The model under review builds one solid part; all positions refer to its coordinate system, in mm. Face numbers are marked on the shaded views. A direction names the side the tool comes from. Coordinates: 2 decimals unless noted, no trailing zeros. Write each loop counter-clockwise with the first axis right and the second up, starting at its lowest first coordinate (ties: lowest second). Pieces come first, ordered by that corner, then holes.
1) For line 1 (Z direction, x = -4.5, y = 3.3); line 2 (X direction, y = 2.3, z = 19.5); line 3 (Z direction, x = -40.5, y = -15.5), list the stretches that pass through material, from the lowest coordinate up.
2) Machinability: for the marked faces 4 and 5, which of the approach directions +Z, -Z, +X, -X, +Y, -Y give a long, thin tool a straight path to every point of the face, cutting with its end or side? Answer none if there is none.
3) For P1, Ø16, axis at x = 5, z = 23, coming from the -Y side; P2, Ø12, axis at x = -50, z = 31, coming from the -Y side, all flat-tipped, find the tip position at first contact; note any pin that passes through.
4) Add section B-B, the plane x = -4.5. State the section outline as (y, z) points, then the cut area to 3 significant figures.
5) Add section A-A, the plane z = 19.5. Give the number of separate pieces and of enclosed holes in the cut face, then the cut area to 3 significant figures.
6) Mouldability with a two-part tool opening along Z and no side actions: class the marked faces 1, 2 and 3 as released by +Z, released by -Z, zero draft, split by the parting line, or undercut.
7) Add section C-C, the plane x = -37. State the section outline as (y, z) points, then the cut area to 3 significant figures.
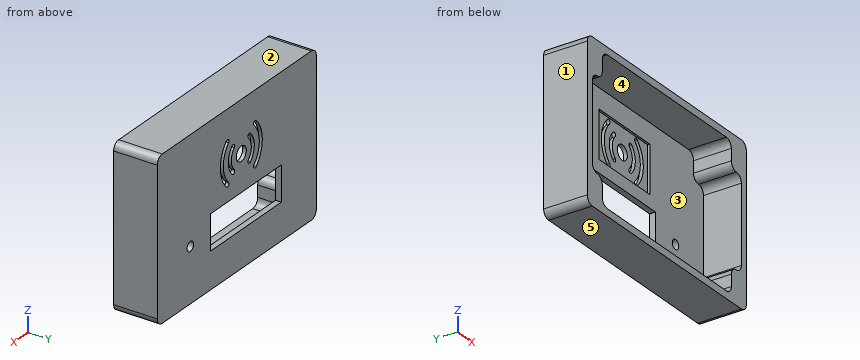
Autodesk Fusion 360 part; units mm, degrees
sketch "Skizze1" plane through (0, 0, 0) normal (0, 1, 0) x (1, 0, 0)
  line L0 (-79.5, 54.5) -> (79.5, 54.5)
  line L1 (79.5, 54.5) -> (79.5, -54.5)
  line L2 (79.5, -54.5) -> (-79.5, -54.5)
  line L3 (-79.5, -54.5) -> (-79.5, 54.5)
  line L4 (-79.5, 54.5) -> (79.5, -54.5) construction
  line L5 (79.5, 54.5) -> (-79.5, -54.5) construction
  dimension "d1" = 109
  dimension "d2" = 159
extrude "Extrusion1" add sketch "Skizze1" along normal blind 4
fillet "Abrundung1" radius 5 4 edges at (-79.5, 2, -54.5) (-79.5, 2, 54.5) (79.5, 2, 54.5) (79.5, 2, -54.5)
sketch "Skizze2" plane through (0, 4, 0) normal (0, 1, 0) x (-1, 0, 0)
  arc A0 (-79.5, -49.5) -> (-74.5, -54.5) centre (-74.5, -49.5) ccw
  line L0 (-74.5, -54.5) -> (74.5, -54.5)
  arc A1 (74.5, -54.5) -> (79.5, -49.5) centre (74.5, -49.5) ccw
  line L1 (79.5, -49.5) -> (79.5, 49.5)
  arc A2 (79.5, 49.5) -> (74.5, 54.5) centre (74.5, 49.5) ccw
  line L2 (74.5, 54.5) -> (-74.5, 54.5)
  arc A3 (-74.5, 54.5) -> (-79.5, 49.5) centre (-74.5, 49.5) ccw
  line L3 (-79.5, 49.5) -> (-79.5, -49.5)
  circle A4 centre (-46.5, -17.5) radius 3.25
  line L4 (44.5, -29.5) -> (-26.5, -29.5)
  line L5 (-26.5, -29.5) -> (-26.5, -5.5)
  line L6 (-26.5, -5.5) -> (44.5, -5.5)
  line L7 (44.5, -5.5) -> (44.5, -29.5)
  circle A5 centre (4.5, 19.5) radius 5
  line L8 (4.5, 19.5) -> (-9.2886, 5.7114) construction
  line L9 (4.5, 19.5) -> (-9.2886, 33.2886) construction
  arc A6 (-10.3492, 4.6508) -> (-8.2279, 6.7721) centre (-9.2886, 5.7114) ccw
  arc A7 (-8.2279, 32.2279) -> (-10.3492, 34.3492) centre (-9.2886, 33.2886) ccw
  arc A8 (-2.5711, 26.5711) -> (-4.6924, 28.6924) centre (-3.6317, 27.6317) ccw
  arc A9 (-4.6924, 10.3076) -> (-2.5711, 12.4289) centre (-3.6317, 11.3683) ccw
  arc A10 (-4.6924, 28.6924) -> (-4.6924, 10.3076) centre (4.5, 19.5) ccw
  arc A11 (-2.5711, 26.5711) -> (-2.5711, 12.4289) centre (4.5, 19.5) ccw
  arc A12 (-8.2279, 32.2279) -> (-8.2279, 6.7721) centre (4.5, 19.5) ccw
  arc A13 (-10.3492, 34.3492) -> (-10.3492, 4.6508) centre (4.5, 19.5) ccw
  line L10 (4.5, 19.5) -> (4.5, 4.5) construction
  arc A14 (19.3492, 34.3492) -> (17.2279, 32.2279) centre (18.2886, 33.2886) ccw
  arc A15 (17.2279, 6.7721) -> (19.3492, 4.6508) centre (18.2886, 5.7114) ccw
  arc A16 (19.3492, 4.6508) -> (19.3492, 34.3492) centre (4.5, 19.5) ccw
  arc A17 (11.5711, 12.4289) -> (13.6924, 10.3076) centre (12.6317, 11.3683) ccw
  arc A18 (11.5711, 12.4289) -> (11.5711, 26.5711) centre (4.5, 19.5) ccw
  arc A19 (13.6924, 28.6924) -> (11.5711, 26.5711) centre (12.6317, 27.6317) ccw
  arc A20 (17.2279, 6.7721) -> (17.2279, 32.2279) centre (4.5, 19.5) ccw
  arc A21 (13.6924, 10.3076) -> (13.6924, 28.6924) centre (4.5, 19.5) ccw
  point P0 (18.2886, 33.2886)
  point P1 (18.2886, 5.7114)
  dimension "d7" = 6.5
  dimension "d8" = 71
  dimension "d9" = 24
  dimension "d10" = 35
  dimension "d11" = 25
  dimension "d12" = 20
  dimension "d13" = 12
  dimension "d14" = 10
  dimension "d15" = 5
  dimension "d16" = 5
  dimension "d17" = 3
  dimension "d18" = 3
  dimension "d21" = 35
  dimension "d22" = 75
  dimension "d23" = 45
extrude "Extrusion2" cut sketch "Skizze2" against normal blind 4 contours A4 | L4 L5 L6 L7 | A5 | A6 A7 A12 A13 | A8 A9 A10 A11 | A14 A15 A16 A20 | A17 A18 A19 A21
sketch "Skizze3" plane through (0, 0, 0) normal (0, -1, 0) x (1, 0, 0)
  line L0 (26.5, -5.5) -> (26.5, -29.5)
  line L1 (26.5, -29.5) -> (-44.5, -29.5)
  line L2 (-44.5, -29.5) -> (-44.5, -5.5)
  line L3 (-44.5, -5.5) -> (26.5, -5.5)
  circle A0 centre (46.5, -17.5) radius 3.25
  arc A1 (74.5, -54.5) -> (79.5, -49.5) centre (74.5, -49.5) ccw
  line L4 (79.5, -49.5) -> (79.5, 49.5)
  arc A2 (79.5, 49.5) -> (74.5, 54.5) centre (74.5, 49.5) ccw
  line L5 (74.5, 54.5) -> (-74.5, 54.5)
  line L6 (-79.5, 49.5) -> (-79.5, -49.5)
  arc A3 (-79.5, -49.5) -> (-74.5, -54.5) centre (-74.5, -49.5) ccw
  line L7 (-74.5, -54.5) -> (74.5, -54.5)
sketch "Skizze4" plane through (0, 0, 0) normal (0, -1, 0) x (1, 0, 0)
  arc A0 (10.3492, 4.6508) -> (10.3492, 34.3492) centre (-4.5, 19.5) ccw
  arc A1 (8.2279, 6.7721) -> (10.3492, 4.6508) centre (9.2886, 5.7114) ccw
  arc A2 (8.2279, 6.7721) -> (8.2279, 32.2279) centre (-4.5, 19.5) ccw
  arc A3 (10.3492, 34.3492) -> (8.2279, 32.2279) centre (9.2886, 33.2886) ccw
  arc A4 (-17.2279, 32.2279) -> (-19.3492, 34.3492) centre (-18.2886, 33.2886) ccw
  arc A5 (-17.2279, 32.2279) -> (-17.2279, 6.7721) centre (-4.5, 19.5) ccw
  arc A6 (-19.3492, 4.6508) -> (-17.2279, 6.7721) centre (-18.2886, 5.7114) ccw
  arc A7 (-19.3492, 34.3492) -> (-19.3492, 4.6508) centre (-4.5, 19.5) ccw
  arc A8 (2.5711, 12.4289) -> (4.6924, 10.3076) centre (3.6317, 11.3683) ccw
  arc A9 (2.5711, 12.4289) -> (2.5711, 26.5711) centre (-4.5, 19.5) ccw
  arc A10 (4.6924, 28.6924) -> (2.5711, 26.5711) centre (3.6317, 27.6317) ccw
  arc A11 (4.6924, 10.3076) -> (4.6924, 28.6924) centre (-4.5, 19.5) ccw
  line L0 (26.5, -5.5) -> (26.5, -29.5)
  line L1 (26.5, -29.5) -> (-44.5, -29.5)
  line L2 (-44.5, -29.5) -> (-44.5, -5.5)
  line L3 (-44.5, -5.5) -> (26.5, -5.5)
  arc A12 (-13.6924, 28.6924) -> (-13.6924, 10.3076) centre (-4.5, 19.5) ccw
  arc A13 (-11.5711, 26.5711) -> (-13.6924, 28.6924) centre (-12.6317, 27.6317) ccw
  arc A14 (-11.5711, 26.5711) -> (-11.5711, 12.4289) centre (-4.5, 19.5) ccw
  arc A15 (-13.6924, 10.3076) -> (-11.5711, 12.4289) centre (-12.6317, 11.3683) ccw
  circle A16 centre (-4.5, 19.5) radius 5
  circle A17 centre (46.5, -17.5) radius 3.25
  arc A18 (74.5, -54.5) -> (79.5, -49.5) centre (74.5, -49.5) ccw
  line L4 (79.5, -49.5) -> (79.5, 49.5)
  arc A19 (79.5, 49.5) -> (74.5, 54.5) centre (74.5, 49.5) ccw
  line L5 (74.5, 54.5) -> (-74.5, 54.5)
  arc A20 (-74.5, 54.5) -> (-79.5, 49.5) centre (-74.5, 49.5) ccw
  line L6 (-79.5, 49.5) -> (-79.5, -49.5)
  arc A21 (-79.5, -49.5) -> (-74.5, -54.5) centre (-74.5, -49.5) ccw
  line L7 (-74.5, -54.5) -> (74.5, -54.5)
  line L8 (-29.75, 35.75) -> (20.75, 35.75)
  line L9 (20.75, 35.75) -> (20.75, 3.25)
  line L10 (20.75, 3.25) -> (-29.75, 3.25)
  line L11 (-29.75, 3.25) -> (-29.75, 35.75)
  line L12 (-29.75, 35.75) -> (20.75, 3.25) construction
  line L13 (20.75, 35.75) -> (-29.75, 3.25) construction
  point P0 (-4.5, 19.5)
  dimension "d50" = 50.5
  dimension "d51" = 32.5
extrude "Extrusion3" cut sketch "Skizze4" against normal blind 1.5 contours L8 L9 L10 L11
sketch "Skizze5" plane through (0, 0, 0) normal (0, -1, 0) x (1, 0, 0)
  line L0 (20.75, 35.75) -> (20.75, 3.25)
  line L1 (20.75, 3.25) -> (-29.75, 3.25)
  line L2 (-29.75, 3.25) -> (-29.75, 35.75)
  line L3 (-29.75, 35.75) -> (20.75, 35.75)
  line L4 (26.5, -5.5) -> (26.5, -29.5)
  line L5 (26.5, -29.5) -> (-44.5, -29.5)
  line L6 (-44.5, -29.5) -> (-44.5, -5.5)
  line L7 (-44.5, -5.5) -> (26.5, -5.5)
  circle A0 centre (46.5, -17.5) radius 3.25
  arc A1 (74.5, -54.5) -> (79.5, -49.5) centre (74.5, -49.5) ccw
  line L8 (79.5, -49.5) -> (79.5, 49.5)
  arc A2 (79.5, 49.5) -> (74.5, 54.5) centre (74.5, 49.5) ccw
  line L9 (74.5, 54.5) -> (-74.5, 54.5)
  arc A3 (-74.5, 54.5) -> (-79.5, 49.5) centre (-74.5, 49.5) ccw
  line L10 (-79.5, 49.5) -> (-79.5, -49.5)
  arc A4 (-79.5, -49.5) -> (-74.5, -54.5) centre (-74.5, -49.5) ccw
  line L11 (-74.5, -54.5) -> (74.5, -54.5)
  line L12 (74.5, 54.5) -> (-74.5, 54.5)
  arc A5 (-74.5, 54.5) -> (-79.5, 49.5) centre (-74.5, 49.5) ccw
  line L13 (-79.5, 49.5) -> (-79.5, -49.5)
  arc A6 (-79.5, -49.5) -> (-74.5, -54.5) centre (-74.5, -49.5) ccw
  line L14 (-74.5, -54.5) -> (74.5, -54.5)
  arc A7 (74.5, -54.5) -> (79.5, -49.5) centre (74.5, -49.5) ccw
  line L15 (79.5, -49.5) -> (79.5, 49.5)
  arc A8 (79.5, 49.5) -> (74.5, 54.5) centre (74.5, 49.5) ccw
  line L16 (-64.5, 49.5) -> (64.5, 49.5)
  line L17 (64.5, 49.5) -> (64.5, 31.5)
  line L18 (64.5, 31.5) -> (74.5, 31.5)
  line L19 (74.5, 31.5) -> (74.5, -31.5)
  line L20 (74.5, -31.5) -> (64.5, -31.5)
  line L21 (64.5, -31.5) -> (64.5, -49.5)
  line L22 (64.5, -49.5) -> (-64.5, -49.5)
  line L23 (-64.5, -49.5) -> (-64.5, -31.5)
  line L24 (-64.5, -31.5) -> (-74.5, -31.5)
  line L25 (-74.5, -31.5) -> (-74.5, 31.5)
  line L26 (-74.5, 31.5) -> (-64.5, 31.5)
  line L27 (-64.5, 31.5) -> (-64.5, 49.5)
  dimension "d54" = 5
  dimension "d55" = 5
  dimension "d56" = 5
  dimension "d57" = 5
  dimension "d58" = 15
  dimension "d59" = 23
extrude "Extrusion4" add sketch "Skizze5" along normal blind 26 contours A1 L8 A2 L9 A3 L10 A4 L11 L12 A5 L13 A6 L14 A7 L15 A8
fillet "Abrundung2" radius 5 12 edges at (64.5, -13, 49.5) (64.5, -13, 31.5) (74.5, -13, 31.5) (64.5, -13, -31.5) (74.5, -13, -31.5) (64.5, -13, -49.5) (-64.5, -13, -49.5) (-64.5, -13, -31.5) (-74.5, -13, -31.5) (-64.5, -13, 31.5) (-74.5, -13, 31.5) (-64.5, -13, 49.5)
equation "d13 = d9 / 2"
equation "d15 = d16"
equation "d17 = d18"
Geometry results:
1. line 1: z = -54.5 to -29.5, -5.5 to 14.5, 24.5 to 54.5
1. line 2: x = -79.5 to -25.5, -22.5 to -17.5, -14.5 to -9.5, 0.5 to 5.5, 8.5 to 13.5, 16.5 to 79.5
1. line 3: z = -54.5 to -49.5, 49.5 to 54.5
2. face 4: -Y
2. face 5: -Z, +X, -X, +Y, -Y
3. P1: stops at y = 1.5
3. P2: stops at y = 0
4. outline: (-26, -54.5) - (4, -54.5) - (4, -29.5) - (0, -29.5) - (0, -49.5) - (-26, -49.5) - close; (-26, 49.5) - (0, 49.5) - (0, 35.75) - (1.5, 35.75) - (1.5, 24.5) - (4, 24.5) - (4, 54.5) - (-26, 54.5) - close; (0, -5.5) - (4, -5.5) - (4, 14.5) - (1.5, 14.5) - (1.5, 3.25) - (0, 3.25) - close
4. area: 526 mm2
5. separate pieces: 6
5. enclosed holes: 0
5. area: 765 mm2
6. face 1: zero draft
6. face 2: released by +Z
6. face 3: undercut
7. outline: (-26, -54.5) - (4, -54.5) - (4, -29.5) - (0, -29.5) - (0, -49.5) - (-26, -49.5) - close; (-26, 49.5) - (0, 49.5) - (0, -5.5) - (4, -5.5) - (4, 54.5) - (-26, 54.5) - close
7. area: 600 mm2
